Here's how the part is built. I have some questions about the finished solid (model axes, mm). Face numbers are marked on the shaded views. Round coordinates to 2 decimals unless told otherwise and drop trailing zeros. One line per item, written item: value. Start each with the question number.
Item 1: For P1, Ø1.6, axis at x = -14.5, z = 5.5, coming from the +Y side; P2, Ø1.5, axis at x = -32.5, z = 5, coming from the -Y side; P3, Ø2.5, axis at x = -10, y = 0, coming from the +Z side, each with a flat end and sliding along its axis, tell me the tip position at first contact or that it passes through.
Item 2: If I drill on line 1 (Y direction, x = 17.5, z = 0.55); line 2 (X direction, y = 0.25, z = 6.5); line 3 (Y direction, x = -12.5, z = 6.25), over which ranges is the centre line in solid material (lowest first)?
Item 3: Thinking about a two-plate mould opening in X: for the marked faces 1 and 2, which applies, released by +X, released by -X, zero draft, split by the parting line, or undercut?
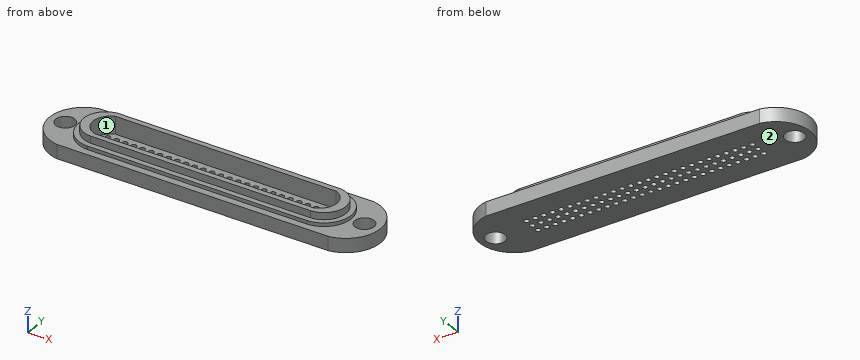
```python
from build123d import *

# Parameters (mm, degrees)
F0_R     = 2.75
F1_DEPTH = 4
F2_DEPTH = 5
F3_DEPTH = 7
F4_DEPTH = 2
F5_R     = 0.75
F5_R_2   = 0.7
F6_DEPTH = 25


with BuildPart() as f1:
    # F0 (on Top) → F1 (new body)
    with BuildSketch(Plane.XY):
        with BuildLine():
            Line((-38.977494, -9.75), (0, -9.75))
            Line((0, -9.75), (38.977494, -9.75))
            ThreePointArc((38.977494, -9.75), (47.498043, -0.167837), (39.370675, 9.75))
            Line((39.370675, 9.75), (0, 9.75))
            Line((0, 9.75), (-39.370675, 9.75))
            ThreePointArc((-39.370675, 9.75), (-47.498043, -0.167837), (-38.977494, -9.75))
        make_face()
        with Locations((-43, 0)):
            Circle(F0_R, mode=Mode.SUBTRACT)
        with BuildLine():
            ThreePointArc((-31.644462, -7.748965), (-39.122501, -0.217996), (-32.104186, 7.743147))
            Line((-32.104186, 7.743147), (-31.961884, 7.75))
            Line((-31.961884, 7.75), (0, 7.75))
            Line((0, 7.75), (31.961884, 7.75))
            Line((31.961884, 7.75), (32.104186, 7.743147))
            ThreePointArc((32.104186, 7.743147), (39.122501, -0.217996), (31.644462, -7.748965))
            Line((31.644462, -7.748965), (31.587565, -7.75))
            Line((31.587565, -7.75), (0.328864, -7.75))
            Line((0.328864, -7.75), (-0.328864, -7.75))
            Line((-0.328864, -7.75), (-31.587565, -7.75))
            Line((-31.587565, -7.75), (-31.644462, -7.748965))
        make_face(mode=Mode.SUBTRACT)
        with Locations((43, 0)):
            Circle(F0_R, mode=Mode.SUBTRACT)
    extrude(amount=F1_DEPTH)

    # F0 (on Top) → F2 (join)
    with BuildSketch(Plane.XY):
        with BuildLine():
            Line((-31.961884, 7.75), (-32.104186, 7.743147))
            ThreePointArc((-32.104186, 7.743147), (-39.122501, -0.217996), (-31.644462, -7.748965))
            Line((-31.644462, -7.748965), (-31.587565, -7.75))
            Line((-31.587565, -7.75), (-0.328864, -7.75))
            Line((-0.328864, -7.75), (0.328864, -7.75))
            Line((0.328864, -7.75), (31.587565, -7.75))
            Line((31.587565, -7.75), (31.644462, -7.748965))
            ThreePointArc((31.644462, -7.748965), (39.122501, -0.217996), (32.104186, 7.743147))
            Line((32.104186, 7.743147), (31.961884, 7.75))
            Line((31.961884, 7.75), (0, 7.75))
            Line((0, 7.75), (-31.961884, 7.75))
        make_face()
        with BuildLine():
            Line((31.587565, -6.25), (-0.328864, -6.25))
            Line((-0.328864, -6.25), (-5.279422, -6.25))
            Line((-5.279422, -6.25), (-31.588749, -6.25))
            ThreePointArc((-31.588749, -6.25), (-37.623142, -0.174144), (-31.960962, 6.25))
            Line((-31.960962, 6.25), (0, 6.25))
            Line((0, 6.25), (31.961884, 6.25))
            ThreePointArc((31.961884, 6.25), (37.62311, -0.175133), (31.587565, -6.25))
        make_face(mode=Mode.SUBTRACT)
    extrude(amount=F2_DEPTH)

    # F0 (on Top) → F3 (join)
    with BuildSketch(Plane.XY):
        with BuildLine():
            Line((-5.279422, -6.25), (-0.328864, -6.25))
            Line((-0.328864, -6.25), (31.587565, -6.25))
            ThreePointArc((31.587565, -6.25), (37.62311, -0.175133), (31.961884, 6.25))
            Line((31.961884, 6.25), (0, 6.25))
            Line((0, 6.25), (-31.960962, 6.25))
            ThreePointArc((-31.960962, 6.25), (-37.623142, -0.174144), (-31.588749, -6.25))
            Line((-31.588749, -6.25), (-5.279422, -6.25))
        make_face()
        with BuildLine():
            Line((31.389172, -4.75), (-0.328864, -4.75))
            Line((-0.328864, -4.75), (-5.279422, -4.75))
            Line((-5.279422, -4.75), (-31.389172, -4.75))
            ThreePointArc((-31.389172, -4.75), (-34.997071, -0.117987), (-31.714512, 4.75))
            Line((-31.714512, 4.75), (0, 4.75))
            Line((0, 4.75), (31.714512, 4.75))
            ThreePointArc((31.714512, 4.75), (34.997071, -0.117987), (31.389172, -4.75))
        make_face(mode=Mode.SUBTRACT)
    extrude(amount=F3_DEPTH)

    # F0 (on Top) → F4 (join)
    with BuildSketch(Plane.XY):
        with BuildLine():
            Line((-5.279422, -4.75), (-0.328864, -4.75))
            Line((-0.328864, -4.75), (31.389172, -4.75))
            ThreePointArc((31.389172, -4.75), (34.997071, -0.117987), (31.714512, 4.75))
            Line((31.714512, 4.75), (0, 4.75))
            Line((0, 4.75), (-31.714512, 4.75))
            ThreePointArc((-31.714512, 4.75), (-34.997071, -0.117987), (-31.389172, -4.75))
            Line((-31.389172, -4.75), (-5.279422, -4.75))
        make_face()
    extrude(amount=F4_DEPTH)

    # F5 (on face) → F6 (cut)
    with BuildSketch(Plane.XY.offset(2)):
        with BuildLine():
            ThreePointArc((0, 0.75), (-0.75, 0), (0, -0.75))
            ThreePointArc((0, -0.75), (0.75, 0), (0, 0.75))
        make_face()
        with BuildLine():
            ThreePointArc((0, 3.25), (-0.75, 2.5), (0, 1.75))
            ThreePointArc((0, 1.75), (0.75, 2.5), (0, 3.25))
        make_face()
        with Locations((2.5, 0)):
            Circle(F5_R)
        with Locations((2.5, 2.5)):
            Circle(F5_R)
        with Locations((5, 0)):
            Circle(F5_R)
        with Locations((5, 2.5)):
            Circle(F5_R)
        with Locations((7.5, 0)):
            Circle(F5_R)
        with Locations((7.5, 2.5)):
            Circle(F5_R)
        with Locations((10, 0)):
            Circle(F5_R)
        with Locations((10, 2.5)):
            Circle(F5_R)
        with Locations((12.5, 0)):
            Circle(F5_R)
        with Locations((12.5, 2.5)):
            Circle(F5_R)
        with Locations((15, 0)):
            Circle(F5_R)
        with Locations((15, 2.5)):
            Circle(F5_R)
        with Locations((17.5, 0)):
            Circle(F5_R)
        with Locations((17.5, 2.5)):
            Circle(F5_R)
        with Locations((20, 0)):
            Circle(F5_R)
        with Locations((20, 2.5)):
            Circle(F5_R)
        with Locations((22.5, 0)):
            Circle(F5_R)
        with Locations((22.5, 2.5)):
            Circle(F5_R)
        with Locations((25, 0)):
            Circle(F5_R)
        with Locations((25, 2.5)):
            Circle(F5_R)
        with Locations((27.5, 0)):
            Circle(F5_R)
        with Locations((27.5, 2.5)):
            Circle(F5_R)
        with Locations((2.5, -2.5)):
            Circle(F5_R)
        with Locations((5, -2.5)):
            Circle(F5_R)
        with Locations((7.5, -2.5)):
            Circle(F5_R)
        with Locations((10, -2.5)):
            Circle(F5_R)
        with Locations((12.5, -2.5)):
            Circle(F5_R)
        with Locations((15, -2.5)):
            Circle(F5_R)
        with Locations((17.5, -2.5)):
            Circle(F5_R)
        with Locations((20, -2.5)):
            Circle(F5_R)
        with Locations((22.5, -2.5)):
            Circle(F5_R)
        with Locations((25, -2.5)):
            Circle(F5_R)
        with Locations((27.5, -2.5)):
            Circle(F5_R)
        with Locations((-12.5, 0)):
            Circle(F5_R)
        with Locations((-17.5, 0)):
            Circle(F5_R)
        with Locations((-7.5, 0)):
            Circle(F5_R)
        with Locations((-5, 0)):
            Circle(F5_R)
        with Locations((-15, 0)):
            Circle(F5_R)
        with Locations((-20, 0)):
            Circle(F5_R)
        with Locations((-10, 0)):
            Circle(F5_R)
        with Locations((-12.5, 2.5)):
            Circle(F5_R)
        with Locations((-10, 2.5)):
            Circle(F5_R)
        with Locations((-7.5, 2.5)):
            Circle(F5_R)
        with Locations((-5, 2.5)):
            Circle(F5_R)
        with Locations((-2.5, 0)):
            Circle(F5_R)
        with Locations((-2.5, 2.5)):
            Circle(F5_R)
        with Locations((-17.5, 2.5)):
            Circle(F5_R)
        with Locations((-15, 2.5)):
            Circle(F5_R)
        with Locations((-20, 2.5)):
            Circle(F5_R)
        with Locations((-27.5, 0)):
            Circle(F5_R)
        with Locations((-22.5, 0)):
            Circle(F5_R)
        with Locations((-25, 0)):
            Circle(F5_R)
        with Locations((-27.5, -2.5)):
            Circle(F5_R)
        with Locations((-25, 2.5)):
            Circle(F5_R)
        with Locations((-22.5, 2.5)):
            Circle(F5_R)
        with Locations((-17.5, -2.5)):
            Circle(F5_R)
        with Locations((-27.5, 2.5)):
            Circle(F5_R)
        with Locations((-20, -2.5)):
            Circle(F5_R)
        with Locations((-22.5, -2.5)):
            Circle(F5_R)
        with Locations((-25, -2.5)):
            Circle(F5_R)
        with Locations((-2.5, -2.5)):
            Circle(F5_R)
        with Locations((-5, -2.5)):
            Circle(F5_R)
        with Locations((-7.5, -2.5)):
            Circle(F5_R)
        with Locations((-10, -2.5)):
            Circle(F5_R)
        with Locations((-12.5, -2.5)):
            Circle(F5_R)
        with Locations((-15, -2.5)):
            Circle(F5_R)
        with Locations((0.020794, -2.485011)):
            Circle(F5_R_2)
        with Locations((-29.956931, 0.036661)):
            Circle(F5_R)
        with Locations((29.956931, 0.036661)):
            Circle(F5_R)
        with Locations((29.949998, 2.5)):
            Circle(F5_R)
        with Locations((32.449998, 2.5)):
            Circle(F5_R)
        with Locations((29.949998, -2.5)):
            Circle(F5_R)
        with Locations((32.449998, 0)):
            Circle(F5_R)
        with Locations((32.449998, -2.5)):
            Circle(F5_R)
        with Locations((-32.466013, 0.00955)):
            Circle(F5_R)
        with Locations((-32.466013, -2.49045)):
            Circle(F5_R)
        with Locations((-29.966013, 2.50955)):
            Circle(F5_R)
        with Locations((-32.466013, 2.50955)):
            Circle(F5_R)
        with Locations((-29.966013, -2.49045)):
            Circle(F5_R)
    extrude(amount=-F6_DEPTH, mode=Mode.SUBTRACT)


solid = f1.part
```
Values follow:
1. P1: stops at y = 7.75
1. P2: stops at y = -7.74
1. P3: stops at z = 2
2. line 1: y = -9.75 to -3.25, -1.75 to -0.75, 0.75 to 1.75, 3.25 to 9.75
2. line 2: x = -37.62 to -35, 35 to 37.62
2. line 3: y = -6.25 to -4.75, 4.75 to 6.25
3. face 1: undercut
3. face 2: zero draft
